Input: dimensioned drawing with shaded views. Units: mm. Origin: part minimum x, y, z. A direction names the side the tool comes from. Round coordinates to 2 decimals unless told otherwise and drop trailing zeros. Order: outer loops, then holes, each group sorted by start corner. A loop starts at its lowest first (then second) coordinate and runs counter-clockwise, first axis right, second up. Notation, with made-up numbers: M -8.75,56.25 L 45.25,56.25 A16 cw 45.25,61.25 Z; hole C -29,53 d7. An arc over 180 degrees is marked long. Answer as CSV lines item,"result". Start each with the question number.
Item 1: First-contact query: P1, Ø5, axis at x = 36, y = 7.5, coming from the +Z side; P2, Ø6, axis at y = 23, z = 5.5, coming from the -X side; P3, Ø10, axis at x = 92, y = 5, coming from the -Z side; P4, Ø2, axis at x = 23, z = 2, coming from the -Y side. Flat tips, straight axial feed; report the tip coordinate or a pass-through.
Item 2: Line query: line 1 (Y direction, x = 10, z = 7.5); line 2 (X direction, y = 22, z = 5.25); line 3 (Y direction, x = 6, z = 2). Output: solid intervals per line, ascending. Write a range as [from, to].
Item 3: Section query D-D on x = 70. Return the cut outline in (y, z), plus the area to 3 significant figures.
Item 4: Section query A-A on y = 22. Return the cut outline in (x, z), plus the area to 3 significant figures.
Item 5: Section query B-B on x = 10. Return the cut outline in (y, z).
Item 6: Set-up query: the marked faces 1, 2, 3 and 4. Return all of +Z, -Z, +X, -X, +Y, -Y with unobstructed straight access to the full face (end or side cutting, diameter ignored); none if empty.
Item 7: Section query C-C on z = 9.5. Return the cut outline in (x, y), plus the area to 3 significant figures.
Item 8: Pull-direction query (Y, two-part tool) for the marked faces 5, 6 and 7; classes: +Y half, -Y half, draft (parallel to the pull), parting line (faces both ways), or undercut.
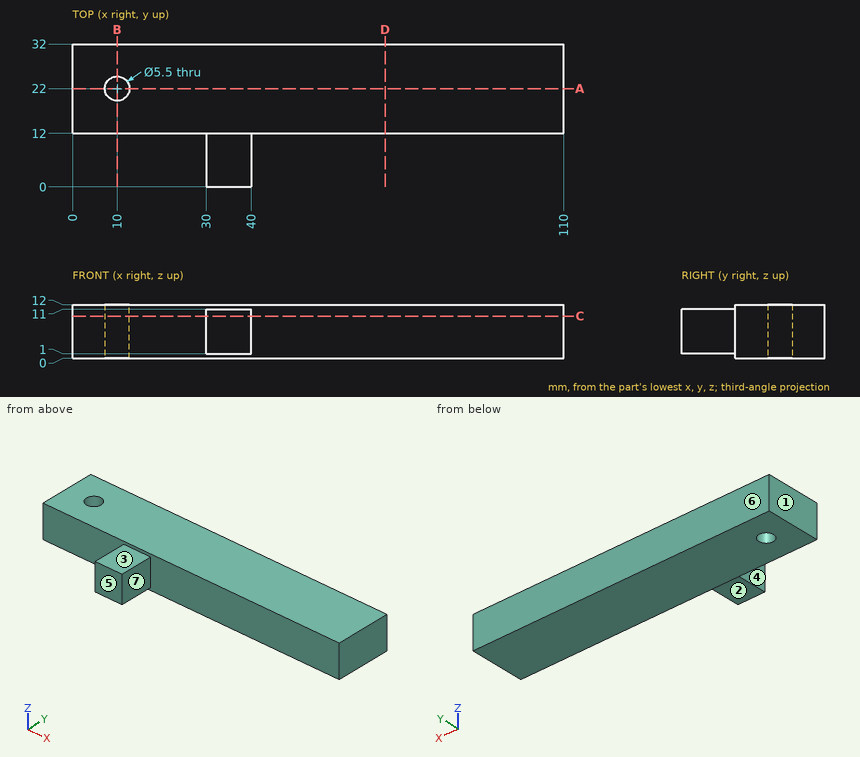
Results:
1,P1,"z = 11"
1,P2,"x = 0"
1,P3,"through"
1,P4,"y = 12"
2,line 1,"[12, 19.25], [24.75, 32]"
2,line 2,"[0, 7.25], [12.75, 110]"
2,line 3,"[12, 32]"
3,outline,"M 12,0 L 32,0 L 32,12 L 12,12 Z"
3,area,"240 mm^2"
4,outline,"M 0,0 L 7.25,0 L 7.25,12 L 0,12 Z; M 12.75,0 L 110,0 L 110,12 L 12.75,12 Z"
4,area,"1,250 mm^2"
5,outline,"M 12,0 L 19.25,0 L 19.25,12 L 12,12 Z; M 24.75,0 L 32,0 L 32,12 L 24.75,12 Z"
6,face 1,"+Z, -Z, -X, +Y, -Y"
6,face 2,"-Z, +X, -X, -Y"
6,face 3,"+Z, +X, -X, -Y"
6,face 4,"+Z, -Z, -X, -Y"
7,outline,"M 0,12 L 30,12 L 30,0 L 40,0 L 40,12 L 110,12 L 110,32 L 0,32 Z; hole C 10,22 d5.5"
7,area,"2,300 mm^2"
8,face 5,"-Y half"
8,face 6,"+Y half"
8,face 7,"draft"
